The drawing under review shows one solid part. Ordinate dimensions are in mm from its lowest x, y, z. A direction names the side the tool comes from. Coordinates: 2 decimals unless noted, no trailing zeros. Write each loop counter-clockwise with the first axis right and the second up, starting at its lowest first coordinate (ties: lowest second). Pieces come first, ordered by that corner, then holes.
1) For P1, Ø0.8, axis at x = 4, z = 4, coming from the -Y side; P2, Ø1.5, axis at y = 7, z = 5, coming from the +X side, all flat-tipped, find the tip position at first contact; note any pin that passes through.
2) For line 1 (Y direction, x = 4.5, z = 5); line 2 (Y direction, x = 2, z = 5.5); line 3 (Z direction, x = 3.75, y = 9.5) (1 decimal), list the stretches that pass through material, from the lowest coordinate up.
3) Add section B-B, the plane y = 1.75. State the section outline as (x, z) points, then the cut area to 3 significant figures.
4) Mouldability with a two-part tool opening along Z and no side actions: class the marked faces 3, 4, 5 and 6 as released by +Z, released by -Z, zero draft, split by the parting line, or undercut.
5) Add section A-A, the plane x = 4. State the section outline as (y, z) points.
6) Add section C-C, the plane y = 7.5. State the section outline as (x, z) points, then the cut area to 3 significant figures.
7) Machinability: for the marked faces 1 and 2, which of the approach directions +Z, -Z, +X, -X, +Y, -Y give a long, thin tool a straight path to every point of the face, cutting with its end or side? Answer none if there is none.
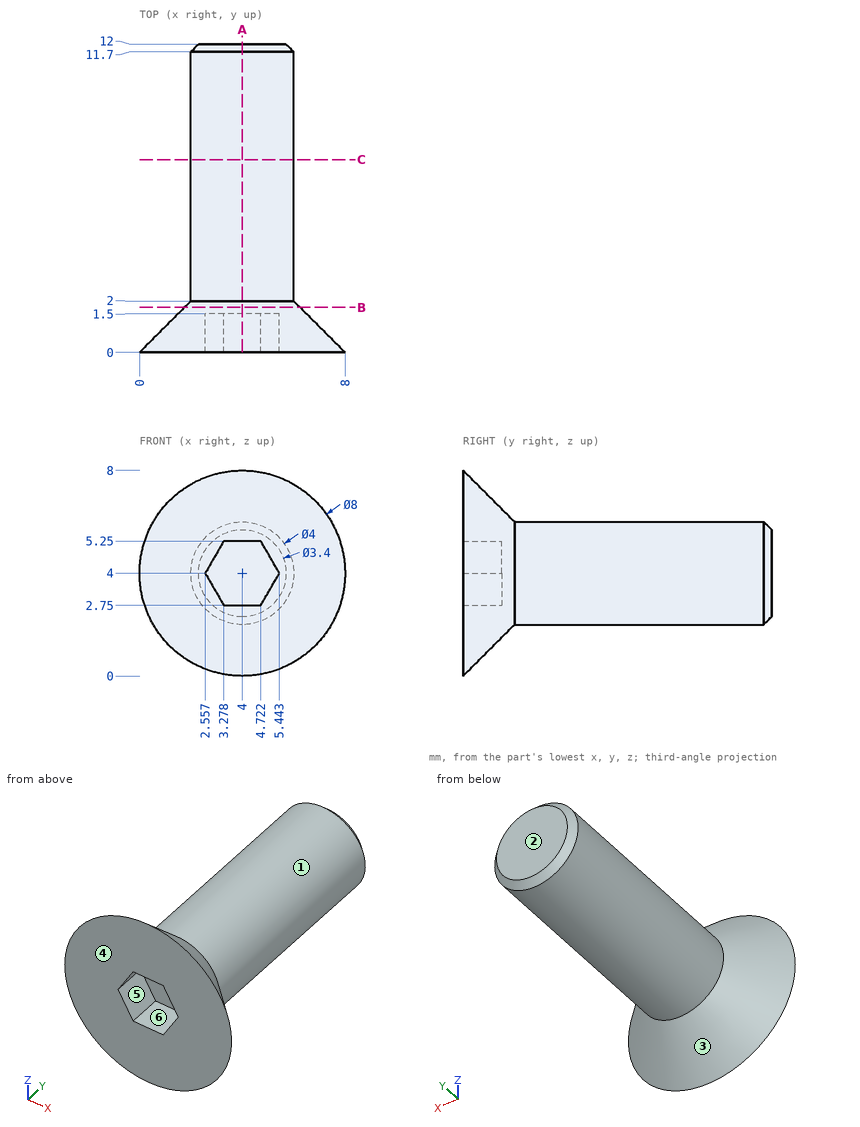
Geometry results:
1. P1: stops at y = 1.5
1. P2: stops at x = 5.98
2. line 1: y = 1.5 to 12
2. line 2: y = 0 to 1.5
2. line 3: z = 2 to 6
3. outline: circle Ø4.5 at (4, 4)
3. area: 15.9 mm2
4. face 3: split by the parting line
4. face 4: zero draft
4. face 5: undercut
4. face 6: undercut
5. outline: (0, 0) - (2, 2) - (11.7, 2) - (12, 2.3) - (12, 5.7) - (11.7, 6) - (2, 6) - (0, 8) - (0, 5.25) - (1.5, 5.25) - (1.5, 2.75) - (0, 2.75) - close
6. outline: circle Ø4 at (4, 4)
6. area: 12.6 mm2
7. face 1: +Y
7. face 2: +Z, -Z, +X, -X, +Y
